Can you work these out from the model? Positions are in its coordinate system, mm. A direction names the side the tool comes from. Round coordinates to 2 decimals unless told otherwise and drop trailing zeros. Write each loop counter-clockwise with the first axis right and the second up, starting at its lowest first coordinate (ties: lowest second). Pieces come first, ordered by that corner, then holes. Notation, with made-up numbers: M -6.75,80.5 L 7.25,80.5 A36 cw 7.25,117.5 Z; hole C 14.25,59 d9. An arc over 180 degrees is marked long. Answer in a Markdown table with one row per item. Add a question column.
(1) If I drill on probe 1 along X at (y, z) = (-4, 2.25); probe 2 along Y at (x, z) = (11.5, 4.5), over which ranges is the centre line in solid material (lowest first)?
(2) Suppose I cut it at C-C, the plane y = -10.5. Write out the boundary of the cut face in (x, z).
(3) Suppose I cut it at A-A, the plane z = 2.5. Write out the boundary of the cut face in (x, y), then the cut area to 3 significant figures.
(4) If we mould it in two halves opening along X, with no side actions, what happens to faces 1 (the face through (0, -13.75, 2)), 2 (the face through (13.75, 0, 2)), 3 (the face through (0, -12, 3))? For each: released by +X, released by -X, zero draft, split by the parting line, or undercut.
(5) For faces 4 (the face through (0, -10, 3)), 5 (the face through (0, 0, -2)), which set-ups out of +Z, -Z, +X, -X, +Y, -Y let a thin tool reach every point of the face, with its end or its side?
(6) Suppose I cut it at B-B, the plane x = -6.75. Write out the boundary of the cut face in (y, z).
from build123d import *

# Parameters (mm, degrees)
F0_W     = 27.5
F0_H     = 27.5
F0_W_2   = 24
F0_H_2   = 24
F0_W_3   = 20
F0_H_3   = 20
F1_DEPTH = 2
F2_DEPTH = 6


with BuildPart() as f1:
    # F0 (on Top) → F1 (new body)
    with BuildSketch(Plane.XY):
        Rectangle(F0_W, F0_H)
        Rectangle(F0_W_2, F0_H_2, mode=Mode.SUBTRACT)
        Rectangle(F0_W_2, F0_H_2)
        Rectangle(F0_W_3, F0_H_3, mode=Mode.SUBTRACT)
        Rectangle(F0_W_3, F0_H_3)
    extrude(amount=-F1_DEPTH)

    # F0 (on Top) → F2 (join)
    with BuildSketch(Plane.XY):
        Rectangle(F0_W, F0_H)
        Rectangle(F0_W_2, F0_H_2, mode=Mode.SUBTRACT)
        Rectangle(F0_W_3, F0_H_3)
    extrude(amount=F2_DEPTH)


solid = f1.part
Calculated:
| question | item | result |
|---|---|---|
| 1 | probe 1 | -13.75 to -12, -10 to 10, 12 to 13.75 |
| 1 | probe 2 | -13.75 to -12, 12 to 13.75 |
| 2 | outline | M -13.75,-2 L 13.75,-2 L 13.75,6 L 12,6 L 12,0 L -12,0 L -12,6 L -13.75,6 Z |
| 3 | outline | M -13.75,-13.75 L 13.75,-13.75 L 13.75,13.75 L -13.75,13.75 Z; M -10,-10 L 10,-10 L 10,10 L -10,10 Z; hole M -12,-12 L 12,-12 L 12,12 L -12,12 Z |
| 3 | area | 580 mm² |
| 4 | face 1 | zero draft |
| 4 | face 2 | released by +X |
| 4 | face 3 | undercut |
| 5 | face 4 | +Z |
| 5 | face 5 | -Z, +X, -X, +Y, -Y |
| 6 | outline | M -13.75,-2 L 13.75,-2 L 13.75,6 L 12,6 L 12,0 L 10,0 L 10,6 L -10,6 L -10,0 L -12,0 L -12,6 L -13.75,6 Z |
